Solid Edge part; units mm, degrees
sketch "Sketch1" plane through (0, 0, 0) normal (0, 0, 1) x (1, 0, 0)
  circle A0 centre (0, 0) radius 5.95
extrude "ExtrudedProtrusion_1" add sketch "Sketch1" along normal blind 5
sketch "Sketch2" plane through (0, 0, 5) normal (0, 0, 1) x (-1, 0, 0)
  circle A0 centre (0, -4) radius 5.95
extrude "ExtrudedProtrusion_5" add sketch "Sketch2" along normal blind 5
sketch "Sketch3" plane through (0, 4, 10) normal (0, 0, 1) x (0, 1, 0)
  circle A0 centre (-2, 3) radius 1.75
  circle A1 centre (-2, -3) radius 1.75
extrude "Cutout1" cut sketch "Sketch3" against normal through all
Read the model definition and answer for the solid it produces. Units are mm, in the model's axes. A direction names the side the tool comes from. Coordinates: 2 decimals unless noted, no trailing zeros. Write each loop counter-clockwise with the first axis right and the second up, starting at its lowest first coordinate (ties: lowest second). Pieces come first, ordered by that corner, then holes. Notation, with made-up numbers: (65, 65.5) -> (109, 65.5) arc R22 cw to (109, 91.5) -> close; hole circle Ø9 at (8.25, 33). An arc over 180 degrees is marked (long way). Return JSON: item names as keys, results as strings.
1. Determine the mould class of faces 4 (the face through (0, 4, 10)), 5 (the face through (-1.45, 2.81, 5.07)), 6 (the face through (3.67, 3.617, 5.07)), 7 (the face through (4.72, 0.38, 7.46)) for opening direction Y: pulls with the +Y half, pulls with the -Y half, needs draft (parallel to the pull), parting line crosses it, or undercut.
Found:
{"face 4": "needs draft", "face 5": "undercut", "face 6": "undercut", "face 7": "parting line crosses it"}
2. Find the intervals of material crossed by line 1 along X through (y, z) = (2, 4.75); line 2 along X through (y, z) = (1, 3.25); line 3 along Z through (x, y) = (4.75, 5), in increasing order. Write a range as from..to.
Found:
{"line 1": "-5.6..-4.75, -1.25..1.25, 4.75..5.6", "line 2": "-5.87..-4.44, -1.56..1.56, 4.44..5.87", "line 3": "5..10"}
3. A cutting plane is placed at D-D (z = 4.25). Determine the outline of the cut face in (x, y), and give its area (3 significant figures).
Found:
{"outline": "circle Ø11.9 at (0, 0); hole circle Ø3.5 at (-3, 2); hole circle Ø3.5 at (3, 2)", "area": "92.0 mm2"}
4. A cutting plane is placed at A-A (y = 0.5). Determine the outline of the cut face in (x, z).
Found:
{"outline": "(-5.93, 0) -> (-3.9, 0) -> (-3.9, 10) -> (-4.81, 10) -> (-4.81, 5) -> (-5.93, 5) -> close; (-2.1, 0) -> (2.1, 0) -> (2.1, 10) -> (-2.1, 10) -> close; (3.9, 0) -> (5.93, 0) -> (5.93, 5) -> (4.81, 5) -> (4.81, 10) -> (3.9, 10) -> close"}
5. Each of these flat-tipped pins is pushed along its axis until it touches: P1, Ø2.5, axis at x = 3, y = 5.5, coming from the -Z side; P2, Ø2, axis at x = -3, y = 2, coming from the -Z side; P3, Ø5, axis at x = -1, z = 1.5, coming from the +Y side. Where does it stop, or does it pass through?
Found:
{"P1": "z = 0", "P2": "through", "P3": "y = 5.95"}
6. A cutting plane is placed at B-B (x = -2). Determine the outline of the cut face in (y, z), and give its area (3 significant figures).
Found:
{"outline": "(-5.6, 0) -> (0.56, 0) -> (0.56, 10) -> (-1.6, 10) -> (-1.6, 5) -> (-5.6, 5) -> close; (3.44, 0) -> (5.6, 0) -> (5.6, 5) -> (9.6, 5) -> (9.6, 10) -> (3.44, 10) -> close", "area": "83.4 mm2"}
7. A cutting plane is placed at C-C (x = 0). Determine the outline of the cut face in (y, z), and give its area (3 significant figures).
Found:
{"outline": "(-5.95, 0) -> (5.95, 0) -> (5.95, 5) -> (9.95, 5) -> (9.95, 10) -> (-1.95, 10) -> (-1.95, 5) -> (-5.95, 5) -> close", "area": "119 mm2"}
8. A tool of negligible diameter and unlimited length cuts with its end or side. For faces 1 (the face through (0, -3, 5)), 2 (the face through (-4.385, -4.021, 2.465)), 3 (the face through (0, 0, 0)), from which of +Z, -Z, +X, -X, +Y, -Y can it reach the whole face along a straight path? Write none if from no direction.
Found:
{"face 1": "+Z, -Y", "face 2": "-Z", "face 3": "-Z, +X, -X, +Y, -Y"}
